```python
from build123d import *

# Parameters (mm, degrees)
SKETCH1_R           = 9
BOSS_EXTRUDE1_DEPTH = 7
BOSS_EXTRUDE2_START = 85
SKETCH2_R           = 9
BOSS_EXTRUDE2_DEPTH = 7
FILLET1_R           = 14
FILLET2_R           = 7


with BuildPart() as part:
    # Sketch1 → Boss-Extrude1 (new body)
    with BuildSketch(Plane(origin=(0, 0, 0), x_dir=(1, 0, 0), z_dir=(0, 1, 0))):
        with BuildLine():
            Line((-19.615045246, 10.5), (-85, 10.5))
            Line((-85, 10.5), (-85, -10.5))
            Line((-85, -10.5), (-19.615045246, -10.5))
            ThreePointArc((-19.615045246, -10.5), (-17.435595774, -11), (-15.692036197, -12.4))
            ThreePointArc((-15.692036197, -12.4), (20, 0), (-15.692036197, 12.4))
            ThreePointArc((-15.692036197, 12.4), (-17.435595774, 11), (-19.615045246, 10.5))
        make_face()
        with Locations(Location((0, 0, 0), (0, 0, 270))):
            Circle(SKETCH1_R, mode=Mode.SUBTRACT)
    extrude(amount=-BOSS_EXTRUDE1_DEPTH)

    # Sketch2 → Boss-Extrude2 (add)
    with BuildSketch(Plane(origin=(0, -33.238764045, -33.238764045), x_dir=(0, -1, 0), z_dir=(-1, 0, 0)).offset(BOSS_EXTRUDE2_START)):
        with BuildLine():
            Line((2.146190709, 43.738764045), (-33.238764045, 43.738764045))
            Line((-33.238764045, 43.738764045), (-33.238764045, 22.738764045))
            Line((-33.238764045, 22.738764045), (2.146190709, 22.738764045))
            ThreePointArc((2.146190709, 22.738764045), (4.325640181, 22.238764045), (6.069199758, 20.838764045))
            ThreePointArc((6.069199758, 20.838764045), (41.761235955, 33.238764045), (6.069199758, 45.638764045))
            ThreePointArc((6.069199758, 45.638764045), (4.325640181, 44.238764045), (2.146190709, 43.738764045))
        make_face()
        with Locations(Location((21.761235955, 33.238764045, 0), (0, 0, 90))):
            Circle(SKETCH2_R, mode=Mode.SUBTRACT)
    extrude(amount=-BOSS_EXTRUDE2_DEPTH)

    # Fillet1
    fillet1_edges = [part.edges().sort_by_distance(p)[0] for p in [
        (-85, 0, 0),
    ]]
    fillet(fillet1_edges, radius=FILLET1_R)

    # Fillet2
    fillet2_edges = [part.edges().sort_by_distance(p)[0] for p in [
        (-78, -7, 0),
    ]]
    fillet(fillet2_edges, radius=FILLET2_R)


solid = part.part
```
Check sheet for the modelled part. Datum: model origin and axes. Units: mm. A direction names the side the tool comes from. Round coordinates to 2 decimals unless told otherwise and drop trailing zeros. Order: outer loops, then holes, each group sorted by start corner. A loop starts at its lowest first (then second) coordinate and runs counter-clockwise, first axis right, second up. Notation, with made-up numbers: (-30, 74) - (13, 74) arc R21 ccw to (13, 96) - close; hole circle Ø2 at (80, 68). An arc over 180 degrees is marked (long way). Answer as CSV lines item,"result". Start each with the question number.
1) Depth check by flat-ended pin: pin 1 (5 mm diameter, centred on y = -30, z = 6.5, fed in from +X); pin 2 (1 mm diameter, centred on x = -44, z = 4.5, fed in from -Y). Enter the tip coordinate at first touch or a pass-through.
2) Section check C-C (z = 0). Record the cut outline in (x, y).
3) Section check B-B (x = 0). Record the cut outline in (y, z), then the cut area to 3 significant figures.
4) Tool access check on faces 5 (the face through (-78, -44, 0)), 6 (the face through (-60, -6, -10.5)), 7 (the face through (-17.46, -3.45, 10.99)), 8 (the face through (-81.549, -37.593, 11.014)), 9 (the face through (-62, -6, 10.5)). Record the directions out of +Z, -Z, +X, -X, +Y, -Y that give a thin tool (end or side, any length) a straight path to the whole face; none if there is none.
5) Section check A-A (z = -16). Record the cut outline in (x, y), then the cut area to 3 significant figures.
6) Draft check along X on faces 1 (the face through (-75.9, -9, 0.1)), 2 (the face through (-17.407, -3.451, -11.014)), 3 (the face through (-26, 0, 0)), 4 (the face through (2.703, -3.451, 8.584)). Enter one of: +X half, -X half, draft (parallel to the pull), parting line (faces both ways), or undercut.
7) Section check D-D (y = -31.5). Record the cut outline in (x, z).
8) Scan lines: probe 1 along Y at (x, z) = (-41, 8.5); probe 2 along X at (y, z) = (-46.5, 15); probe 3 along Y at (x, z) = (-82, 0). Record each from-to range of solid material in increasing order.
Determined:
1,pin 1,"x = -78"
1,pin 2,"y = -7"
2,outline,"(-85, -75) - (-78, -75) - (-78, -64) - (-85, -64) - close; (-85, -46) - (-78, -46) - (-78, -14) arc R7 cw to (-71, -7) - (-9, -7) - (-9, 0) - (-71, 0) arc R14 ccw to (-85, -14) - close; (9, -7) - (20, -7) - (20, 0) - (9, 0) - close"
3,outline,"(-7, -20) - (0, -20) - (0, -9) - (-7, -9) - close; (-7, 9) - (0, 9) - (0, 20) - (-7, 20) - close"
3,area,"154 mm^2"
4,face 5,"+Z, -Z, +X, -Y"
4,face 6,"-Z, -X, +Y"
4,face 7,"+Z, -X, +Y, -Y"
4,face 8,"+Z, +X, -X, +Y"
4,face 9,"+Z, -X, +Y"
5,outline,"(-85, -67) - (-78, -67) - (-78, -43) - (-85, -43) - close; (-12, -7) - (12, -7) - (12, 0) - (-12, 0) - close"
5,area,"336 mm^2"
6,face 1,"+X half"
6,face 2,"-X half"
6,face 3,"draft"
6,face 4,"undercut"
7,outline,"(-85, -10.5) - (-78, -10.5) - (-78, 10.5) - (-85, 10.5) - close"
8,probe 1,"-7 to 0"
8,probe 2,"-85 to -78"
8,probe 3,"-75 to -64, -46 to -5.34"
